```python
from build123d import *

# Parameters (mm, degrees)
SKETCH1_W           = 60
SKETCH1_H           = 30
SKETCH1_W_2         = 3
SKETCH1_H_2         = 20
SKETCH1_W_3         = 30
SKETCH1_H_3         = 3
BOSS_EXTRUDE1_DEPTH = 1.5


with BuildPart() as part:
    # Sketch1 → Boss-Extrude1 (new body, symmetric)
    with BuildSketch(Plane.XY):
        Rectangle(SKETCH1_W, SKETCH1_H)
        with Locations((-27, 0)):
            Rectangle(SKETCH1_W_2, SKETCH1_H_2, mode=Mode.SUBTRACT)
        with Locations((27, 0)):
            Rectangle(SKETCH1_W_2, SKETCH1_H_2, mode=Mode.SUBTRACT)
        with Locations((0, 12.5)):
            Rectangle(SKETCH1_W_3, SKETCH1_H_3, mode=Mode.SUBTRACT)
        with Locations((0, -12.5)):
            Rectangle(SKETCH1_W_3, SKETCH1_H_3, mode=Mode.SUBTRACT)
    extrude(amount=BOSS_EXTRUDE1_DEPTH, both=True)


solid = part.part
```
Check sheet for the modelled part. Datum: model origin and axes. Units: mm. A direction names the side the tool comes from. Give positions to 0.01 mm unless a question says otherwise; leave off trailing zeros. Write each loop counter-clockwise with the first axis right and the second up, starting at its lowest first coordinate (ties: lowest second). Pieces come first, ordered by that corner, then holes. Notation, with made-up numbers: (67.5, -19.5) - (119.5, -19.5) arc R7 cw to (119.5, -8.5) - close; hole circle Ø2 at (48, -25.75). An arc over 180 degrees is marked (long way). Answer as a JSON object with one key per item and string values. Group by question number.
1) Thickness scan on probe 1 along X at (y, z) = (-8.75, 0.95); probe 2 along Y at (x, z) = (0, -0.85); probe 3 along Y at (x, z) = (-26.5, 0.95). Record the ranges inside material, lowest first. Write a range as from..to.
2) Sectioned sample at A-A (y = 8). Record the cut outline in (x, z).
3) Sectioned sample at B-B (z = -0.75). Record the cut outline in (x, y), then the cut area to 3 significant figures.
4) Access from +Z, -Z, +X, -X, +Y, -Y to the whole of each face (thin tool, end or side, straight path). Record for faces 5 (the face through (0, 14, 0)), 6 (the face through (0, 0, -1.5)).
5) Sectioned sample at C-C (x = 11). Record the cut outline in (y, z), then the cut area to 3 significant figures.
6) Release check for a two-part mould opening along Y. For faces 1 (the face through (27, 10, 0)), 2 (the face through (0, -15, 0)), 3 (the face through (28.5, 0, 0)), 4 (the face through (0, 15, 0)) record: pulls with the +Y half, pulls with the -Y half, needs draft (parallel to the pull), parting line crosses it, or undercut.
Geometry results:
{
 "1": {"probe 1": "x = -30..-28.5, -25.5..25.5, 28.5..30", "probe 2": "y = -15..-14, -11..11, 14..15", "probe 3": "y = -15..-10, 10..15"},
 "2": {"outline": "(-30, -1.5) - (-28.5, -1.5) - (-28.5, 1.5) - (-30, 1.5) - close; (-25.5, -1.5) - (25.5, -1.5) - (25.5, 1.5) - (-25.5, 1.5) - close; (28.5, -1.5) - (30, -1.5) - (30, 1.5) - (28.5, 1.5) - close"},
 "3": {"outline": "(-30, -15) - (30, -15) - (30, 15) - (-30, 15) - close; hole (-28.5, -10) - (-25.5, -10) - (-25.5, 10) - (-28.5, 10) - close; hole (-15, -14) - (15, -14) - (15, -11) - (-15, -11) - close; hole (-15, 11) - (15, 11) - (15, 14) - (-15, 14) - close; hole (25.5, -10) - (28.5, -10) - (28.5, 10) - (25.5, 10) - close", "area": "1,500 mm^2"},
 "4": {"face 5": "+Z, -Z", "face 6": "-Z, +X, -X, +Y, -Y"},
 "5": {"outline": "(-15, -1.5) - (-14, -1.5) - (-14, 1.5) - (-15, 1.5) - close; (-11, -1.5) - (11, -1.5) - (11, 1.5) - (-11, 1.5) - close; (14, -1.5) - (15, -1.5) - (15, 1.5) - (14, 1.5) - close", "area": "72.0 mm^2"},
 "6": {"face 1": "undercut", "face 2": "pulls with the -Y half", "face 3": "undercut", "face 4": "pulls with the +Y half"}
}
